Geometry check sheet. Reference: the model listing, model coordinates, mm. Face numbers are marked on the shaded views. Round coordinates to 2 decimals unless told otherwise and drop trailing zeros. Loops run counter-clockwise (first coordinate to the right, second up) from the corner with the lowest first, then second, coordinate; pieces in that order, holes last. Notation, with made-up numbers: M 41,32 L 100,32 A21 cw 100,56 Z; hole C -25.5,-26 d11. An arc over 180 degrees is marked long. Write item = value, one per line.
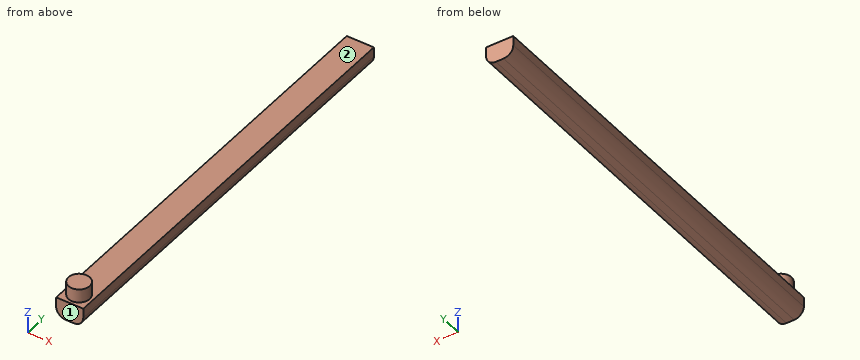
from build123d import *

# Parameters (mm, degrees)
SKETCH1_W           = 7
SKETCH1_H           = 110
BOSS_EXTRUDE1_DEPTH = 5
FILLET4_R           = 2.5
SKETCH2_R           = 2.75
BOSS_EXTRUDE2_DEPTH = 3.5


with BuildPart() as part:
    # Sketch1 → Boss-Extrude1 (new body)
    with BuildSketch(Plane.XY):
        with Locations((3.5, 55)):
            Rectangle(SKETCH1_W, SKETCH1_H)
    extrude(amount=BOSS_EXTRUDE1_DEPTH)

    # Fillet4
    fillet4_edges = [part.edges().sort_by_distance(p)[0] for p in [
        (7, 55, 0),
        (0, 55, 0),
    ]]
    fillet(fillet4_edges, radius=FILLET4_R)

    # Sketch2 → Boss-Extrude2 (add)
    with BuildSketch(Plane.XY.offset(5)):
        with Locations((3.5, 3.548899595)):
            Circle(SKETCH2_R)
    extrude(amount=BOSS_EXTRUDE2_DEPTH)


solid = part.part
(1) Sectioned sample at C-C on z = 6. Record the cut outline in (x, y), then the cut area to 3 significant figures.
Result set:
outline = C 3.5,3.55 d5.5
area = 23.8 mm2
(2) Sectioned sample at A-A on x = 3.5. Record the cut outline in (y, z), then the cut area to 3 significant figures.
Result set:
outline = M 0,0 L 110,0 L 110,5 L 6.3,5 L 6.3,8.5 L 0.8,8.5 L 0.8,5 L 0,5 Z
area = 569 mm2
(3) Release check for a two-part mould opening along Z. For the marked faces 1 and 2 record: released by +Z, released by -Z, zero draft, split by the parting line, or undercut.
Result set:
face_1 = zero draft
face_2 = released by +Z
(4) Sectioned sample at B-B on y = 60.5. Record the cut outline in (x, z).
Result set:
outline = M 0,2.5 A2.5 ccw 2.5,0 L 4.5,0 A2.5 ccw 7,2.5 L 7,5 L 0,5 Z
(5) Material ranges on line 1 along Z through (x, y) = (4.75, 36); line 2 along X through (y, z) = (96.5, 2.25); line 3 along Y through (x, z) = (1.25, 7), recorded low to high. Write a range as from..to.
Result set:
line_1 = 0.01..5
line_2 = 0.01..6.99
line_3 = 1.97..5.13
